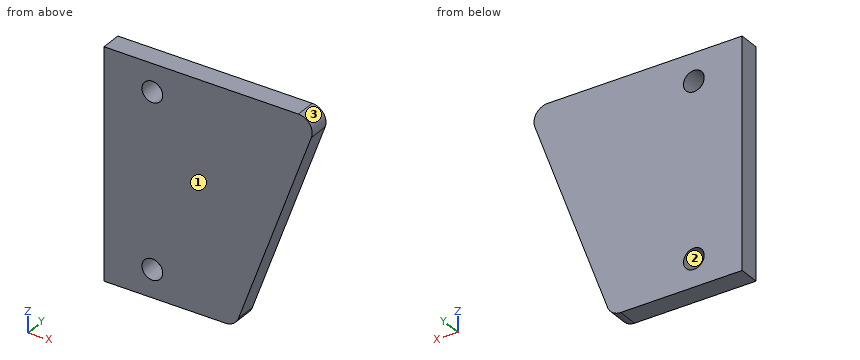
Autodesk Inventor part; units mm, degrees
ref_plane "YZ Plane" through (0, 0, 0) normal (1, 0, 0) x (0, 1, 0)
ref_plane "XZ Plane" through (0, 0, 0) normal (0, 1, 0) x (-1, 0, 0)
ref_plane "XY Plane" through (0, 0, 0) normal (0, 0, 1) x (1, 0, 0)
sketch "Sketch1" plane through (0, 0, 0) normal (0, 1, 0) x (-1, 0, 0)
  line L0 (1.9014, 11.5388) -> (1.9014, -21.4612)
  line L1 (1.9014, -21.4612) -> (-17.0986, -21.4612)
  line L2 (-17.0986, -21.4612) -> (-29.1096, 11.5388)
  line L3 (-29.1096, 11.5388) -> (1.9014, 11.5388)
  line L4 (-17.0986, -21.4612) -> (-17.0986, 11.5388) construction
  point P0 (0, 0)
  dimension "d1" = 33
  dimension "d2" = 20
  dimension "d22" = 19
extrude "Extrusion1" add sketch "Sketch1" along normal blind 3
sketch "Sketch3" plane through (0, 0, 0) normal (0, -1, 0) x (1, 0, 0)
  line L0 (29.1096, 11.5388) -> (-1.9014, 11.5388)
  line L1 (-1.9014, 11.5388) -> (-1.9014, -21.4612)
  line L2 (-1.9014, -21.4612) -> (17.0986, -21.4612)
  point P0 (0, 0)
  point P1 (5.0986, 7.5388)
  point P2 (5.0986, -17.4612)
  dimension "d5" = 4
  dimension "d6" = 4
  dimension "d19" = 7
  dimension "d21" = 7
hole "Hole1" at (5.0986, 0, 7.5388) at (5.0986, 0, -17.4612) direction (0, 1, 0) diameter 3 end through all
fillet "Fillet1" radius 2 1 edges at (29.1096, 1.5, 11.5388)
fillet "Fillet2" radius 2 1 edges at (17.0986, 1.5, -21.4612)
properties part number "k2_feet"
Check sheet for the modelled part. Datum: model origin and axes. Units: mm. Face numbers are marked on the shaded views. Give positions to 0.01 mm unless a question says otherwise; leave off trailing zeros. Loops run counter-clockwise (first coordinate to the right, second up) from the corner with the lowest first, then second, coordinate; pieces in that order, holes last. Notation, with made-up numbers: M -30.75,50.5 L 27.25,50.5 A11 cw 27.25,67.5 Z; hole C -17,0 d4. An arc over 180 degrees is marked long. Answer as a JSON object with one key per item and string values. Group by question number.
Q1. Cross-section at B-B on z = -17.5. Record the cut outline in (x, y).
Q2. Cross-section at A-A on y = 1.5. Record the cut outline in (x, z), then the cut area to 3 significant figures.
Q3. Cross-section at C-C on x = 23.5. Record the cut outline in (y, z), then the cut area to 3 significant figures.
Q4. Release check for a two-part mould opening along X. For the marked faces 1, 2 and 3 record: released by +X, released by -X, zero draft, split by the parting line, or undercut.
Q5. Cross-section at D-D on z = -12. Record the cut outline in (x, y).
Q6. Material ranges on line 1 along X through (y, z) = (2.35, -17); line 2 along X through (y, z) = (1.7, 8.5); line 3 along X through (y, z) = (1.85, -9.5), recorded low to high. Write a range as [from, to].
Evaluation:
{
 "1": {"outline": "M -1.9,0 L 3.6,0 L 3.6,3 L -1.9,3 Z; M 6.6,0 L 18.54,0 L 18.54,3 L 6.6,3 Z"},
 "2": {"outline": "M -1.9,-21.46 L 15.7,-21.46 A2 ccw 17.58,-20.15 L 28.13,8.85 A2 ccw 26.25,11.54 L -1.9,11.54 Z; hole C 5.1,-17.46 d3; hole C 5.1,7.54 d3", "area": "809 mm2"},
 "3": {"outline": "M 0,-3.87 L 3,-3.87 L 3,11.54 L 0,11.54 Z", "area": "46.2 mm2"},
 "4": {"face 1": "zero draft", "face 2": "undercut", "face 3": "released by +X"},
 "5": {"outline": "M -1.9,0 L 20.54,0 L 20.54,3 L -1.9,3 Z"},
 "6": {"line 1": "x = [-1.9, 3.67], [6.53, 18.72]", "line 2": "x = [-1.9, 3.95], [6.25, 28]", "line 3": "x = [-1.9, 21.45]"}
}
